Work out the finished part from the listing and answer in its coordinate system (mm). Round coordinates to 2 decimals unless told otherwise and drop trailing zeros. Put each result on its own line as item: value.
Autodesk Inventor part; units mm, degrees
ref_plane "YZ Plane" through (0, 0, 0) normal (1, 0, 0) x (0, 1, 0)
ref_plane "XZ Plane" through (0, 0, 0) normal (0, 1, 0) x (-1, 0, 0)
ref_plane "XY Plane" through (0, 0, 0) normal (0, 0, 1) x (1, 0, 0)
sketch "Foam Scheme" plane through (0, 0, 0) normal (0, 1, 0) x (-1, 0, 0)
  line L0 (599.5, -94) -> (-599.5, -94)
  line L1 (-599.5, -94) -> (-599.5, 94)
  line L2 (-599.5, 94) -> (599.5, 94)
  line L3 (599.5, 94) -> (599.5, -94)
  circle A0 centre (577.5, -72) radius 9.5
  circle A1 centre (522.5, -72) radius 9.5
  circle A2 centre (467.5, -72) radius 9.5
  circle A3 centre (412.5, -72) radius 9.5
  circle A4 centre (357.5, -72) radius 9.5
  circle A5 centre (302.5, -72) radius 9.5
  circle A6 centre (247.5, -72) radius 9.5
  circle A7 centre (192.5, -72) radius 9.5
  circle A8 centre (137.5, -72) radius 9.5
  circle A9 centre (82.5, -72) radius 9.5
  circle A10 centre (27.5, -72) radius 9.5
  circle A11 centre (-27.5, -72) radius 9.5
  circle A12 centre (-82.5, -72) radius 9.5
  circle A13 centre (-137.5, -72) radius 9.5
  circle A14 centre (-192.5, -72) radius 9.5
  circle A15 centre (-247.5, -72) radius 9.5
  circle A16 centre (-302.5, -72) radius 9.5
  circle A17 centre (-357.5, -72) radius 9.5
  circle A18 centre (577.5, 72) radius 9.5
  circle A19 centre (522.5, 72) radius 9.5
  circle A20 centre (467.5, 72) radius 9.5
  circle A21 centre (412.5, 72) radius 9.5
  circle A22 centre (357.5, 72) radius 9.5
  circle A23 centre (302.5, 72) radius 9.5
  circle A24 centre (247.5, 72) radius 9.5
  circle A25 centre (192.5, 72) radius 9.5
  circle A26 centre (137.5, 72) radius 9.5
  circle A27 centre (82.5, 72) radius 9.5
  circle A28 centre (27.5, 72) radius 9.5
  circle A29 centre (-27.5, 72) radius 9.5
  circle A30 centre (-82.5, 72) radius 9.5
  circle A31 centre (-137.5, 72) radius 9.5
  circle A32 centre (-192.5, 72) radius 9.5
  circle A33 centre (-247.5, 72) radius 9.5
  circle A34 centre (-302.5, 72) radius 9.5
  circle A35 centre (-357.5, 72) radius 9.5
  circle A36 centre (-412.5, -72) radius 9.5
  circle A37 centre (-412.5, 72) radius 9.5
  circle A38 centre (-467.5, -72) radius 9.5
  circle A39 centre (-467.5, 72) radius 9.5
  circle A40 centre (-522.5, -72) radius 9.5
  circle A41 centre (-522.5, 72) radius 9.5
  circle A42 centre (-577.5, -72) radius 9.5
  circle A43 centre (-577.5, 72) radius 9.5
  point P0 (0, 0)
  dimension "d0" = 1199
  dimension "d1" = 599.5
  dimension "d2" = 188
  dimension "d3" = 94
  dimension "d4" = 19
  dimension "d5" = 22
  dimension "d6" = 22
  dimension "d9" = 55
  dimension "d12" = 144
extrude "Foam Body" add sketch "Foam Scheme" along normal blind 1.5
properties part number "Foam NPS 10" material "Rubber, Silicone"
1) For a pull along X with two mould halves and no side action, classify faces 1 (the flat face through (8, 1.5, 1)), 2 (the cylindrical face through (238.439, 0.74, -74.854)) as pulls with the +X half, pulls with the -X half, needs draft (parallel to the pull), parting line crosses it, or undercut.
Findings below:
face 1: needs draft
face 2: undercut
2) Straight lines are drawn through the part: L1, parallel to Z at x = -194.5, y = 0.95; L2, parallel to Z at x = 467.5, y = 0.8. For each, find the intervals that lie inside material, in ascending order. Write a range as from..to.
Findings below:
L1: z = -94..-81.29, -62.71..62.71, 81.29..94
L2: z = -94..-81.5, -62.5..62.5, 81.5..94
3) A cutting plane is placed at A-A on y = 0.4. Give the number of separate pieces and of enclosed holes in the cut face, then the cut area to 3 significant figures.
Findings below:
separate pieces: 1
enclosed holes: 44
area: 213,000 mm2
